from build123d import *

# Parameters (mm, degrees)
F1_DEPTH = 19.05
F3_DEPTH = 8.4666582
F5_DEPTH = 9.525
F6_W     = 94.742
F6_H     = 19.05
F7_DEPTH = 19.05


# Not quite as in the source:
# - a feature names something its author has since deleted; it is built from what else it names


with BuildPart() as f1:
    # F0 (on Top) → F1 (new body)
    with BuildSketch(Plane.XY):
        with BuildLine():
            Line((732.4377516272, 429.8118038565), (732.4377516272, -265.5463867273))
            ThreePointArc((732.4377516272, -265.5463867273), (767.5922703415, -310.3140075425), (819.4192408881, -286.7779674454))
            Line((819.4192408881, -286.7779674454), (819.4192408881, -229.1199674454))
            Line((819.4192408881, -229.1199674454), (1159.4623036636, -98.9686407408))
            Line((1159.4623036636, -98.9686407408), (1178.6487772739, -128.0367093729))
            Line((1178.6487772739, -128.0367093729), (1189.3036458742, -145.3996676047))
            ThreePointArc((1189.3036458742, -145.3996676047), (1254.3589120262, -165.180351508), (1280.8355912672, -102.5508970465))
            Line((1280.8355912672, -102.5508970465), (881.2480453078, 396.8848219998))
            ThreePointArc((881.2480453078, 396.8848219998), (878.9075846932, 401.4943033077), (878.5980767553, 406.6546597539))
            Line((878.5980767553, 406.6546597539), (902.2401524871, 568.497452094))
            ThreePointArc((902.2401524871, 568.497452094), (903.8120375637, 573.0182606597), (906.9455405898, 576.6362285378))
            Line((906.9455405898, 576.6362285378), (941.9003890149, 604.1852707886))
            Line((941.9003890149, 604.1852707886), (899.3018677789, 723.8279303566))
            Line((899.3018677789, 723.8279303566), (891.7270738587, 721.1309406639))
            Line((891.7270738587, 721.1309406639), (888.532184766, 730.1041401315))
            Line((888.532184766, 730.1041401315), (557.8398737201, 612.361827435))
            Line((557.8398737201, 612.361827435), (561.0347628128, 603.3886279674))
            Line((561.0347628128, 603.3886279674), (540.3738890749, 596.0323666485))
            Line((540.3738890749, 596.0323666485), (579.8650741531, 488.7713005475))
            ThreePointArc((579.8650741531, 488.7713005475), (586.4584656719, 481.6292642269), (596.1708798397, 481.2413137672))
            Line((596.1708798397, 481.2413137672), (715.3498421741, 525.1204082985))
            ThreePointArc((715.3498421741, 525.1204082985), (727.0028583004, 523.6192401995), (732.4377516272, 513.202512065))
            Line((732.4377516272, 513.202512065), (732.4377516272, 429.8118038565))
        make_face()
        with BuildLine():
            ThreePointArc((847.6172180507, -123.0333171416), (832.579476833, -121.3659760987), (825.2142352601, -108.1498153983))
            Line((825.2142352601, -108.1498153983), (812.2279623998, 291.9047427935))
            ThreePointArc((812.2279623998, 291.9047427935), (820.3847868922, 304.1789193457), (834.6503380579, 300.4798321914))
            Line((834.6503380579, 300.4798321914), (1091.877202569, -6.0938706764))
            ThreePointArc((1091.877202569, -6.0938706764), (1095.2114543488, -20.8476640537), (1085.1310970041, -32.1249886369))
            Line((1085.1310970041, -32.1249886369), (847.6172180507, -123.0333171416))
        make_face(mode=Mode.SUBTRACT)
    extrude(amount=F1_DEPTH)

    # F2 (on face) → F3 (cut)
    with BuildSketch(Plane.XY.offset(19.05)):
        with BuildLine():
            ThreePointArc((838.451528287, -152.2525984903), (831.9027765287, -166.0430988586), (845.6932768971, -172.5918506169))
            Line((845.6932768971, -172.5918506169), (1132.8356598603, -70.3553996504))
            ThreePointArc((1132.8356598603, -70.3553996504), (1139.3844116185, -56.564899282), (1125.5939112501, -50.0161475238))
            Line((1125.5939112501, -50.0161475238), (838.451528287, -152.2525984903))
        make_face()
    extrude(amount=-F3_DEPTH, mode=Mode.SUBTRACT)

    # F4 (on face) → F5 (cut)
    with BuildSketch(Plane.XY.offset(19.05)):
        Polygon((579.7007303012, 517.0436017545), (586.2609025716, 498.618632181), (926.4367371726, 619.7375338049), (930.6009060633, 621.2201775171), (924.161381266, 639.3062953154), (919.9972123753, 637.8236516032), (891.8491444715, 716.8806143331), (890.4923506062, 720.6913200061), (891.7270738587, 721.1309406639), (888.532184766, 730.1041401315), (869.645537074, 723.3795883228), (874.197220032, 710.5956831823), (902.2246404628, 631.8775722275), align=None)
    extrude(amount=-F5_DEPTH, mode=Mode.SUBTRACT)

    # F6 (on face) → F7 (cut)
    with BuildSketch(Plane(origin=(730.9119602838, 584.7866009261, 0), x_dir=(-0.6247321984, 0.7808390873, 0), z_dir=(0.7808390873, 0.6247321984, 0))):
        with Locations((-357.880134458, 9.525)):
            Rectangle(F6_W, F6_H)
        with Locations((-584.981534458, 9.525)):
            Rectangle(F6_W, F6_H)
    extrude(amount=-F7_DEPTH, mode=Mode.SUBTRACT)


solid = f1.part
Could you check a few things on this model? Use its own coordinates, in mm. A direction names the side the tool comes from. Coordinates: 2 decimals unless noted, no trailing zeros. Write each loop counter-clockwise with the first axis right and the second up, starting at its lowest first coordinate (ties: lowest second). Pieces come first, ordered by that corner, then holes. Notation, with made-up numbers: (-21.75, -34.5) - (31.25, -34.5) arc R20 ccw to (31.25, -10.5) - close; hole circle Ø7 at (83.25, 88.5). An arc over 180 degrees is marked (long way). Write item = value, one per line.
1) Suppose I cut it at D-D on x = 787. Please give me the cut outline in (y, z) (3 decimals), plus the area to 3 significant figures.
Result set:
outline = (-310.841, 0) - (693.954, 0) - (693.954, 19.05) - (590.852, 19.05) - (590.852, 9.525) - (570.091, 9.525) - (570.091, 19.05) - (-310.841, 19.05) - close
area = 18,900 mm2
2) We'd pull the mould along X, two halves only. Please class faces 6 (the flat face through (743.22, 575.264, 14.354)), 7 (the cylindrical face through (766.76, -310.103, 9.392)), 8 (the flat face through (725.501, 672.057, 9.392)), 9 (the flat face through (793, 589, 9.525)): +X half, -X half, draft (parallel to the pull), parting line (faces both ways), or undercut.
Result set:
face_6 = undercut
face_7 = parting line
face_8 = -X half
face_9 = undercut
3) Suppose I cut it at B-B on x = 637. Please give me the cut outline in (y, z) (3 decimals).
Result set:
outline = (496.274, 0) - (640.547, 0) - (640.547, 19.05) - (537.445, 19.05) - (537.445, 9.525) - (516.684, 9.525) - (516.684, 19.05) - (496.274, 19.05) - close
4) Please list where these lines run through material, in increasing order: line 1 (X direction, y = -239, z = 11.5); line 2 (Y direction, x = 1079.5, z = 6.5); line 3 (Y direction, x = 994.5, z = 11.75). Write a range as [from, to].
Result set:
line_1 = [732.44, 819.42]
line_2 = [-129.57, -34.28], [8.66, 118.6]
line_3 = [-162.11, -119.61], [-96.69, -66.81], [109.96, 255.33]
5) Will these pins go through, and if not, where does the flat tip stop? pin 1 Ø1.5 at (y, z) = (542, 17) entering from +X; pin 2 Ø5.5 at (y, z) = (-245.5, 10) entering from +X; pin 3 Ø1.5 at (y, z) = (217.5, 6) entering from +X.
Result set:
pin_1 = 898.48
pin_2 = 819.42
pin_3 = 1025.37
6) Suppose I cut it at C-C on z = 14.5. State how many separate pieces and enclosed holes the cut face has, plus the area to 3 significant figures.
Result set:
separate_pieces = 1
enclosed_holes = 2
area = 212,000 mm2
7) For faces 1 (the flat face through (890.254, 486.443, 9.392)), 2 (the flat face through (1026.01, 215.95, 9.39)), 3 (the flat face through (940.03, 292.92, 9.66)), 4 (the flat face through (654.926, 502.874, 9.392)), 5 (the flat face through (987.25, -122.19, 14.88)), which set-ups out of +Z, -Z, +X, -X, +Y, -Y let a thin tool reach every point of the face, with its end or its side?
Result set:
face_1 = +Z, -Z, +X
face_2 = +Z, -Z, +X, +Y
face_3 = +Z, -Z
face_4 = +Z, -Z, -Y
face_5 = +Z
8) Suppose I cut it at A-A on y = 14.5. Please give me the cut outline in (x, z).
Result set:
outline = (732.44, 0) - (821.23, 0) - (821.23, 19.05) - (732.44, 19.05) - close; (1074.6, 0) - (1187.19, 0) - (1187.19, 19.05) - (1074.6, 19.05) - close
